Verification items for the finished model (mm, model axes). A direction names the side the tool comes from. Round coordinates to 2 decimals unless told otherwise and drop trailing zeros. Loops run counter-clockwise (first coordinate to the right, second up) from the corner with the lowest first, then second, coordinate; pieces in that order, holes last. Notation, with made-up numbers: M 48.25,75 L 80.25,75 A18 cw 80.25,79 Z; hole C 88.5,17 d5. An arc over 180 degrees is marked long. One line per item, written item: value.
from build123d import *

# Parameters (mm, degrees)
BOSS_EXTRUDE1_DEPTH = 50
SKETCH2_R           = 20
BOSS_EXTRUDE2_DEPTH = 30
CUT_EXTRUDE1_START  = -20
CUT_EXTRUDE1_DEPTH  = 20
SKETCH4_W           = 30
SKETCH4_H           = 28
CUT_EXTRUDE2_DEPTH  = 23


with BuildPart() as part:
    # Sketch1 → Boss-Extrude1 (new body)
    with BuildSketch(Plane.XY):
        Polygon((14.59247247, 21.522973704), (-45.40752753, 21.522973704), (-63.40752753, -17.477026296), (-63.40752753, -32.477026296), (-35.40752753, -32.477026296), (-25.40752753, -12.477026296), (-5.40752753, -12.477026296), (4.59247247, -32.477026296), (32.59247247, -32.477026296), (32.59247247, -17.477026296), align=None)
    extrude(amount=BOSS_EXTRUDE1_DEPTH)

    # Sketch2 → Boss-Extrude2 (add)
    with BuildSketch(Plane(origin=(0, 21.522973704, 0), x_dir=(1, 0, 0), z_dir=(0, 1, 0))):
        with Locations(Location((-15.40752753, -25, 0), (0, 0, 270))):
            Circle(SKETCH2_R)
    extrude(amount=BOSS_EXTRUDE2_DEPTH)

    # Sketch3 → Cut-Extrude1 (cut)
    with BuildSketch(Plane(origin=(0, 51.522973704, 0), x_dir=(1, 0, 0), z_dir=(0, 1, 0)).offset(CUT_EXTRUDE1_START)):
        with BuildLine():
            Line((-7.40752753, -25), (-7.40752753, -6.66969722))
            ThreePointArc((-7.40752753, -6.66969722), (-15.40752753, -5), (-23.40752753, -6.66969722))
            Line((-23.40752753, -6.66969722), (-23.40752753, -43.33030278))
            ThreePointArc((-23.40752753, -43.33030278), (-15.40752753, -45), (-7.40752753, -43.33030278))
            Line((-7.40752753, -43.33030278), (-7.40752753, -25))
        make_face()
    extrude(amount=CUT_EXTRUDE1_DEPTH, mode=Mode.SUBTRACT)

    # Sketch4 → Cut-Extrude2 (cut)
    with BuildSketch(Plane.ZY.offset(63.40752753)):
        with Locations((25, 7.522973704)):
            Rectangle(SKETCH4_W, SKETCH4_H)
    cut_extrude2 = extrude(amount=-CUT_EXTRUDE2_DEPTH, mode=Mode.SUBTRACT)

    # Mirror1: Cut-Extrude2 across plane
    add(cut_extrude2.mirror(Plane(origin=(-15.40752753, 0, 0), x_dir=(0, 0, 1), z_dir=(1, 0, 0))), mode=Mode.SUBTRACT)


solid = part.part
(1) Sectioned sample at A-A on y = -25. Enter the section's corners in (x, z), and give its area (3 significant figures).
Completed:
outline: M -63.41,0 L -31.67,0 L -31.67,50 L -63.41,50 Z; M 0.85,0 L 32.59,0 L 32.59,50 L 0.85,50 Z
area: 3,170 mm^2
(2) Sectioned sample at C-C on z = 25. Enter the section's corners in (x, y).
Completed:
outline: M -63.41,-32.48 L -35.41,-32.48 L -25.41,-12.48 L -5.41,-12.48 L 4.59,-32.48 L 32.59,-32.48 L 32.59,-17.48 L 27.52,-6.48 L 9.59,-6.48 L 9.59,21.52 L 4.59,21.52 L 4.59,51.52 L -7.41,51.52 L -7.41,31.52 L -23.41,31.52 L -23.41,51.52 L -35.41,51.52 L -35.41,21.52 L -40.41,21.52 L -40.41,-6.48 L -58.33,-6.48 L -63.41,-17.48 Z
(3) Sectioned sample at D-D on y = -10.5. Enter the section's corners in (x, z), and give its area (3 significant figures).
Completed:
outline: M -60.19,0 L 29.37,0 L 29.37,50 L -60.19,50 Z
area: 4,480 mm^2
(4) Thickness scan on L1, parallel to Z at x = -44, y = 16; L2, parallel to Y at x = -49, z = 34; L3, parallel to Y at x = -39.5, z = 44.5. Record the ranges inside material, lowest first. Write a range as from..to.
Completed:
L1: z = 0..10, 40..50
L2: y = -32.48..-6.48
L3: y = -32.48..21.52
(5) Mould release check, pull along Z, two halves, no side actions. Record for faces 4 (the face through (-1.89, 36.31, 10.26)), 5 (the face through (-16, -5, 0)), 6 (the face through (32.592, -25, 25)), 7 (the face through (-40.408, 8, 25)): +Z half, -Z half, draft (parallel to the pull), parting line (faces both ways), or undercut.
Completed:
face 4: parting line
face 5: -Z half
face 6: draft
face 7: undercut
(6) Sectioned sample at B-B on x = 12. Enter the section's corners in (y, z), and give its area (3 significant figures).
Completed:
outline: M -32.48,0 L 21.52,0 L 21.52,10 L -6.48,10 L -6.48,40 L 21.52,40 L 21.52,50 L -32.48,50 Z
area: 1,860 mm^2
(7) Tool access check on faces 1 (the face through (-48, 4, 10)), 2 (the face through (5, 21.523, 25)), 3 (the face through (-23.408, 41, 25)). Record the directions out of +Z, -Z, +X, -X, +Y, -Y that give a thin tool (end or side, any length) a straight path to the whole face; none if there is none.
Completed:
face 1: -X, +Y
face 2: +Y
face 3: +Z, -Z, +Y
(8) Depth check by flat-ended pin: pin 1 Ø22.5 at (y, z) = (9, 26.5) entering from +X; pin 2 Ø19.5 at (x, y) = (21, 9) entering from -Z; pin 3 Ø8 at (x, z) = (-13, 26.5) entering from +Y; pin 4 Ø9 at (x, z) = (-47, 19) entering from +Y. Enter the tip coordinate at first touch or a pass-through.
Completed:
pin 1: stops at x = 9.59
pin 2: stops at z = 0
pin 3: stops at y = 31.52
pin 4: stops at y = -6.48
